Autodesk Inventor part; units mm, degrees
ref_plane "YZ Plane" through (0, 0, 0) normal (1, 0, 0) x (0, 1, 0)
ref_plane "XZ Plane" through (0, 0, 0) normal (0, 1, 0) x (-1, 0, 0)
ref_plane "XY Plane" through (0, 0, 0) normal (0, 0, 1) x (1, 0, 0)
sketch "Sketch1" plane through (0, 0, 0) normal (0, 0, 1) x (1, 0, 0)
  line L0 (-27.94, 0) -> (27.94, 0)
  line L1 (-27.94, 0) -> (-27.94, 76.2)
  line L2 (-27.94, 76.2) -> (-27.94, 81.28)
  line L3 (-27.94, 81.28) -> (27.94, 81.28)
  line L4 (27.94, 81.28) -> (27.94, 0)
  line L5 (-27.94, 76.2) -> (27.94, 76.2)
  line L6 (0, 0) -> (0, 3.5814)
  line L7 (0, 3.5814) -> (-10.16, 3.5814)
  line L8 (-10.16, 3.5814) -> (10.16, 3.5814)
  circle A0 centre (-10.16, 3.5814) radius 1.524
  circle A1 centre (10.16, 3.5814) radius 1.524
  line L9 (0, 76.2) -> (0, 81.28)
  line L10 (0, 76.2) -> (-5.08, 76.2)
  line L11 (-5.08, 76.2) -> (-5.08, 81.28)
  line L12 (0, 76.2) -> (5.08, 76.2)
  line L13 (5.08, 76.2) -> (5.08, 81.28)
  dimension "d0" = 55.88
  dimension "d1" = 76.2
  dimension "d2" = 5.08
  dimension "d3" = 3.5814
  dimension "d4" = 10.16
  dimension "d5" = 20.32
  dimension "d6" = 3.048
  dimension "d7" = 3.048
  dimension "d8" = 5.08
extrude "Extrusion1" add sketch "Sketch1" along normal blind 3.175 contours L1 L5 L4 L0 | L2 L3 L11 L5 | L5 L13 L3 L4
sketch "Sketch2" plane through (0, 0, 3.175) normal (0, 0, 1) x (1, 0, 0)
  line L0 (-27.94, 81.28) -> (-27.94, 0)
  line L1 (3.4628, 9.8032) -> (-34.29, 119.2864)
  line L2 (-34.29, 119.2864) -> (-34.29, 0)
  line L3 (0, 0) -> (0, 76.2)
  line L4 (5.08, 76.2) -> (-5.08, 76.2)
  line L5 (-3.4628, 9.8032) -> (34.29, 119.2864)
  line L6 (27.94, 0) -> (27.94, 81.28)
  line L7 (27.94, 81.28) -> (5.08, 81.28)
  line L8 (5.08, 81.28) -> (5.08, 76.2)
  line L9 (5.08, 76.2) -> (-5.08, 76.2)
  line L10 (-5.08, 76.2) -> (-5.08, 81.28)
  line L11 (-5.08, 81.28) -> (-27.94, 81.28)
  line L12 (-27.94, 81.28) -> (-27.94, 0)
  line L13 (-27.94, 0) -> (27.94, 0)
  circle A0 centre (-10.16, 3.5814) radius 1.524
  circle A1 centre (10.16, 3.5814) radius 1.524
  line L14 (0, 0) -> (0, 0.254)
  line L15 (-5.08, 81.28) -> (-27.94, 81.28)
  line L16 (0, 0.254) -> (-27.94, 81.28)
  line L17 (0, 0.254) -> (27.94, 81.28)
  point P0 (6.0051, 2.0643)
  point P1 (-6.0051, 2.0643)
  point P2 (21.1843, 81.28)
  point P3 (0, 19.8454)
  point P4 (-21.1843, 81.28)
  dimension "d15" = 0.254
extrude "Extrusion2" cut sketch "Sketch2" against normal blind 1.5875 contours L11 L1 L5 L16 | L5 L3 L16 | L5 L7 L17 L1 | L1 L17 L3 | A0 | A1
fillet "Fillet1" radius 3.175 8 edges at (-13.1322, 81.28, 3.175) (13.1322, 81.28, 3.175) (27.94, 40.64, 3.175) (-27.94, 40.64, 3.175) (-5.08, 78.74, 3.175) (0, 76.2, 3.175) (5.08, 78.74, 3.175) (0, 0, 3.175)
sketch "Sketch3" plane through (0, 0, 1.5875) normal (0, 0, 1) x (1, 0, 0)
  line L0 (0.0591, 0.4254) -> (-0.0591, 0.4254)
  line L1 (27.5146, 80.0464) -> (0.0591, 0.4254)
  line L2 (27.5146, 80.8546) -> (27.5146, 80.0464)
  line L3 (21.0377, 80.8546) -> (27.5146, 80.8546)
  line L4 (0, 19.8454) -> (21.0377, 80.8546)
  line L5 (-21.0377, 80.8546) -> (0, 19.8454)
  line L6 (-27.5146, 80.8546) -> (-21.0377, 80.8546)
  line L7 (-27.5146, 80.0464) -> (-27.5146, 80.8546)
  line L8 (-0.0591, 0.4254) -> (-27.5146, 80.0464)
  circle A0 centre (-24.2761, 78.105) radius 1.524
  line L9 (-27.5146, 80.8546) -> (-27.94, 81.28)
  line L10 (-27.5146, 80.8546) -> (-21.0377, 80.8546)
  line L11 (-21.0377, 80.8546) -> (-20.0895, 78.105)
  line L12 (-20.0895, 78.105) -> (-8.255, 78.105)
  line L13 (-8.255, 78.105) -> (-5.08, 81.28)
  line L14 (-5.08, 81.28) -> (-27.94, 81.28)
  line L15 (-27.94, 81.28) -> (-27.94, 0)
  line L16 (5.08, 76.2) -> (-5.08, 76.2)
  line L17 (0, 76.2) -> (0, 83.5529)
  circle A1 centre (24.2761, 78.105) radius 1.524
  line L18 (-1.0072, 3.175) -> (-8.6912, 3.175)
  line L19 (-1.0072, 3.175) -> (-24.765, 72.0725)
  line L20 (-24.765, 3.175) -> (-24.765, 72.0725)
  line L21 (-11.6288, 3.175) -> (-24.765, 3.175)
  arc A2 (-8.6912, 3.175) -> (-11.6288, 3.175) centre (-10.16, 3.5814) ccw
  line L22 (8.6912, 3.175) -> (1.0072, 3.175)
  arc A3 (11.6288, 3.175) -> (8.6912, 3.175) centre (10.16, 3.5814) ccw
  line L23 (24.765, 3.175) -> (11.6288, 3.175)
  line L24 (24.765, 72.0725) -> (24.765, 3.175)
  line L25 (24.765, 72.0725) -> (1.0072, 3.175)
  point P0 (0, 0)
  point P1 (-24.2761, 80.8546)
  dimension "d16" = 3.048
  dimension "d17" = 3.175
  dimension "d21" = 74.5236
  dimension "d22" = 14.1161
extrude "Extrusion3" cut sketch "Sketch3" against normal blind 25.4 contours A0 | A1
sketch "Sketch4" plane through (0, 0, 3.175) normal (0, 0, 1) x (1, 0, 0)
  line L0 (-1.0072, 3.175) -> (-8.6912, 3.175)
  line L1 (-1.0072, 3.175) -> (-24.765, 72.0725)
  line L2 (-24.765, 3.175) -> (-24.765, 72.0725)
  line L3 (-11.6288, 3.175) -> (-24.765, 3.175)
  arc A0 (-8.6912, 3.175) -> (-11.6288, 3.175) centre (-10.16, 3.5814) ccw
  line L4 (8.6912, 3.175) -> (1.0072, 3.175)
  arc A1 (11.6288, 3.175) -> (8.6912, 3.175) centre (10.16, 3.5814) ccw
  line L5 (24.765, 3.175) -> (11.6288, 3.175)
  line L6 (24.765, 72.0725) -> (24.765, 3.175)
  line L7 (24.765, 72.0725) -> (1.0072, 3.175)
  circle A2 centre (-10.16, 3.5814) radius 1.524
  circle A3 centre (-10.16, 3.5814) radius 2.5
  arc A4 (11.6288, 3.175) -> (8.6912, 3.175) centre (10.16, 3.5814) ccw
  circle A5 centre (10.16, 3.5814) radius 2.5
  point P0 (0, 0)
  point P1 (12.6267, 3.175)
  point P2 (7.6933, 3.175)
  dimension "d23" = 5
  dimension "d24" = 5
extrude "Extrusion4" cut sketch "Sketch4" against normal blind 1.5875 contours A3 L3 A2 L0 | L0 A0 L3 A3 | A2 A0 | A1 L5 A5 L4 | L4 A5 L5 A1
properties part number "holo - laser battery backing"
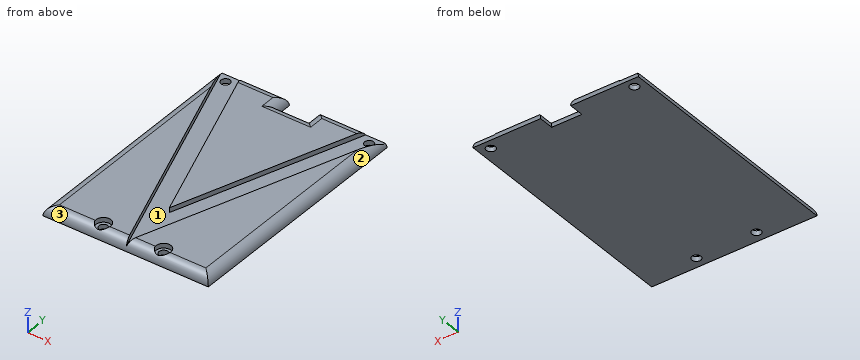
Can you work these out from the model? Positions are in its coordinate system, mm. Face numbers are marked on the shaded views. Give positions to 0.01 mm unless a question says otherwise; leave off trailing zeros. Order: outer loops, then holes, each group sorted by start corner. A loop starts at its lowest first (then second) coordinate and runs counter-clockwise, first axis right, second up. Notation, with made-up numbers: (77, -29) - (126, -29) arc R27 cw to (126, -1) - close; hole circle Ø11 at (61, -21). An arc over 180 degrees is marked (long way). Use a Markdown table: item, result. Add a question column.
Q1. If we mould it in two halves opening along Y, with no side actions, what happens to the marked faces 1, 2 and 3? For each: released by +Y, released by -Y, zero draft, split by the parting line, or undercut.
Q2. If we section it at A-A on z = 0.9: Write out the boundary of the cut face in (x, y) (3 decimals), plus the area to 3 significant figures.
Q3. I'm going to push flat-ended pins straight in: pin 1 (2.5 mm diameter, centred on x = 10.16, y = 3.58, fed in from -Z); pin 2 (3 mm diameter, centred on x = 19, y = 69, fed in from +Z); pin 3 (1.5 mm diameter, centred on x = 5, z = 1, fed in from +Y). Where does each tip first touch, or does it pass through?
Q4. Please list where these lines run through material, in increasing order: line 1 along X through (y, z) = (4, 1.5); line 2 along X through (y, z) = (30, 1.95); line 3 along Z through (x, y) = (-20.5, 62.5).
Answers follow:
| question | item | result |
|---|---|---|
| 1 | face 1 | undercut |
| 1 | face 2 | zero draft |
| 1 | face 3 | released by -Y |
| 2 | outline | (-27.81, 0.13) - (27.81, 0.13) - (27.81, 81.15) - (5.21, 81.15) - (5.21, 76.07) - (-5.21, 76.07) - (-5.21, 81.15) - (-27.81, 81.15) - close; hole circle Ø3.048 at (-24.276, 78.105); hole circle Ø3.048 at (-10.16, 3.581); hole circle Ø3.048 at (10.16, 3.581); hole circle Ø3.048 at (24.276, 78.105) |
| 2 | area | 4,420 mm^2 |
| 3 | pin 1 | passes through |
| 3 | pin 2 | stops at z = 1.59 |
| 3 | pin 3 | stops at y = 81.27 |
| 4 | line 1 | x = -27.56 to -11.63, -8.69 to 8.69, 11.63 to 27.56 |
| 4 | line 2 | x = -27.27 to -10.26, -3.5 to 3.5, 10.26 to 27.27 |
| 4 | line 3 | z = 0 to 1.59 |
